Can you work these out from the model? Positions are in its coordinate system, mm. A direction names the side the tool comes from. Round coordinates to 2 decimals unless told otherwise and drop trailing zeros. Loops run counter-clockwise (first coordinate to the right, second up) from the corner with the lowest first, then second, coordinate; pieces in that order, holes last.
from build123d import *

# Parameters (mm, degrees)
SKETCH1_W            = 35
SKETCH1_H            = 35
BOSS_EXTRUDE1_DEPTH  = 3
BOSS_EXTRUDE2_DEPTH  = 35
SKETCH6_W            = 35
SKETCH6_H            = 38
BOSS_EXTRUDE8_DEPTH  = 2
SKETCH7_W            = 35
SKETCH7_H            = 38
BOSS_EXTRUDE9_DEPTH  = 2
SKETCH8_R            = 1.4
CUT_EXTRUDE1_DEPTH   = 10
SKETCH9_W            = 1
SKETCH9_H            = 35
BOSS_EXTRUDE10_DEPTH = 2
SKETCH10_W           = 3.4
SKETCH10_H           = 2
BOSS_EXTRUDE11_DEPTH = 35
BOSS_EXTRUDE12_DEPTH = 35


with BuildPart() as part:
    # Sketch1 → Boss-Extrude1 (new body)
    with BuildSketch(Plane(origin=(0, 0, 0), x_dir=(1, 0, 0), z_dir=(0, 1, 0))):
        with Locations((-17.5, 17.5)):
            Rectangle(SKETCH1_W, SKETCH1_H)
    extrude(amount=BOSS_EXTRUDE1_DEPTH)

    # Sketch2 → Boss-Extrude2 (add)
    with BuildSketch(Plane(origin=(0, 3, 0), x_dir=(1, 0, 0), z_dir=(0, 1, 0))):
        Polygon((-35, 33.6), (-1.4, 0), (0, 0), (0, 1.428427125), (-33.571572875, 35), (-35, 35), align=None)
    extrude(amount=BOSS_EXTRUDE2_DEPTH)

    # Sketch6 → Boss-Extrude8 (add)
    with BuildSketch(Plane(origin=(0, 0, 0), x_dir=(0, 0, -1), z_dir=(1, 0, 0))):
        with Locations((17.5, 19)):
            Rectangle(SKETCH6_W, SKETCH6_H)
    extrude(amount=BOSS_EXTRUDE8_DEPTH)

    # Sketch7 → Boss-Extrude9 (add)
    with BuildSketch(Plane.ZY.offset(35)):
        with Locations((-17.5, 19)):
            Rectangle(SKETCH7_W, SKETCH7_H)
    extrude(amount=BOSS_EXTRUDE9_DEPTH)

    # Sketch8 → Cut-Extrude1 (cut)
    with BuildSketch(Plane.XZ):
        with Locations((-17.5, -6.5)):
            Circle(SKETCH8_R)
        with Locations((-17.5, -28.5)):
            Circle(SKETCH8_R)
    extrude(amount=-CUT_EXTRUDE1_DEPTH, mode=Mode.SUBTRACT)

    # Sketch9 → Boss-Extrude10 (add)
    with BuildSketch(Plane(origin=(0, 38, 0), x_dir=(1, 0, 0), z_dir=(0, 1, 0))):
        with Locations((-36.5, 17.5)):
            Rectangle(SKETCH9_W, SKETCH9_H)
        with Locations((1.5, 17.5)):
            Rectangle(SKETCH9_W, SKETCH9_H)
    extrude(amount=BOSS_EXTRUDE10_DEPTH)

    # Sketch10 → Boss-Extrude11 (add)
    with BuildSketch(Plane.XY):
        with Locations((-35.3, 41)):
            Rectangle(SKETCH10_W, SKETCH10_H)
        with Locations((0.3, 41)):
            Rectangle(SKETCH10_W, SKETCH10_H)
    extrude(amount=-BOSS_EXTRUDE11_DEPTH)

    # Sketch11 → Boss-Extrude12 (add)
    with BuildSketch(Plane.XY):
        Polygon((-37, 42), (-38, 41), (-38, 36), (-37, 31.101020514), align=None)
        Polygon((2, 42), (3, 41), (3, 36), (2, 31.101020514), align=None)
    extrude(amount=-BOSS_EXTRUDE12_DEPTH)


solid = part.part
(1) For faces 4 (the flat face through (-37, 15, -17)), 5 (the flat face through (0, 40, -17)), 6 (the flat face through (0, 21, -18)), 7 (the flat face through (-1.4, 41, -17)), which set-ups out of +Z, -Z, +X, -X, +Y, -Y let a thin tool reach every point of the face, with its end or its side?
Worked answers:
face 4: +Z, -Z, -X, -Y
face 5: +Z, -Z
face 6: -Z
face 7: +Z, -Z, +Y
(2) If we mould it in two halves opening along Y, with no side actions, what happens to faces 1 (the flat face through (-35, 21, -17)), 2 (the flat face through (-35, 42, -17)), 3 (the flat face through (-38, 39, -17))? For each: released by +Y, released by -Y, zero draft, split by the parting line, or undercut.
Worked answers:
face 1: undercut
face 2: released by +Y
face 3: zero draft
(3) Will these pins go through, and if not, where does the flat tip stop? P1, Ø17, axis at x = -14, z = -20.5, coming from the +Y side; P2, Ø12, axis at x = -9, y = 36, coming from the -Z side; P3, Ø5, axis at x = -22.5, z = -8, coming from the +Y side.
Worked answers:
P1: stops at y = 38
P2: stops at z = -16.43
P3: stops at y = 3
(4) If we section it at A-A, the plane x = -17.5: List the corners of the cut face in (y, z) for me, then the cut area to 3 significant figures.
Worked answers:
outline: (0, -35) - (3, -35) - (3, -29.9) - (0, -29.9) - close; (0, -27.1) - (3, -27.1) - (3, -18.93) - (38, -18.93) - (38, -16.1) - (3, -16.1) - (3, -7.9) - (0, -7.9) - close; (0, -5.1) - (3, -5.1) - (3, 0) - (0, 0) - close
area: 187 mm2
(5) If I drill on line 1 (Z direction, x = -17.5, y = 1.8); line 2 (X direction, y = 33, z = -13.5); line 3 (X direction, y = 26, z = -13), over which ranges is the centre line in solid material (lowest first)?
Worked answers:
line 1: z = -35 to -29.9, -27.1 to -7.9, -5.1 to 0
line 2: x = -37.39 to -35, -14.9 to -12.07, 0 to 2.39
line 3: x = -37 to -35, -14.4 to -11.57, 0 to 2
(6) If we section it at D-D, the plane z = -19.5: List the corners of the cut face in (x, y) for me.
Worked answers:
outline: (-38, 36) - (-37, 31.1) - (-37, 0) - (2, 0) - (2, 31.1) - (3, 36) - (3, 41) - (2, 42) - (-1.4, 42) - (-1.4, 40) - (1, 40) - (1, 38) - (0, 38) - (0, 3) - (-18.07, 3) - (-18.07, 38) - (-20.9, 38) - (-20.9, 3) - (-35, 3) - (-35, 38) - (-36, 38) - (-36, 40) - (-33.6, 40) - (-33.6, 42) - (-37, 42) - (-38, 41) - close
(7) If we section it at B-B, the plane y = 29.5: List the corners of the cut face in (x, z) for me, then the cut area to 3 significant figures.
Worked answers:
outline: (-37, -35) - (-33.57, -35) - (0, -1.43) - (0, -35) - (2, -35) - (2, 0) - (-1.4, 0) - (-35, -33.6) - (-35, 0) - (-37, 0) - close
area: 237 mm2
